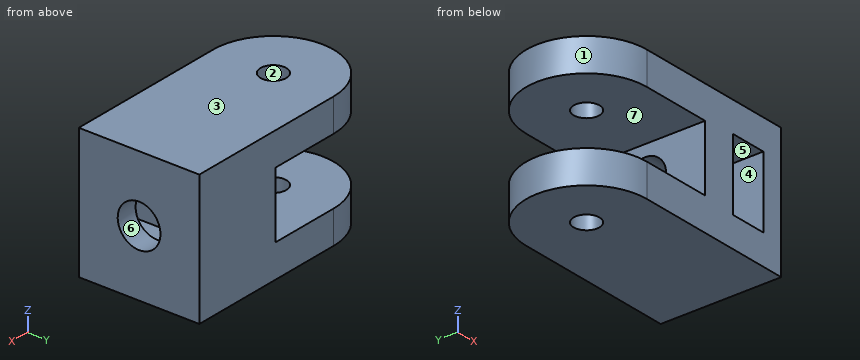
```python
from build123d import *

# Parameters (mm, degrees)
BOSS_EXTRUDE1_DEPTH            = 24
SKETCH2_W                      = 30.110806601
SKETCH2_H                      = 12
CUT_EXTRUDE1_DEPTH             = 45.271887242
CUT_EXTRUDE2_DEPTH             = 6.8
F_7_8_7_8_DIAMETER_HOLE1_D     = 7.8
F_7_8_7_8_DIAMETER_HOLE1_DEPTH = 6.2
F_7_8_7_8_DIAMETER_HOLE2_D     = 7.8
F_4_7_4_7_DIAMETER_HOLE1_D     = 4.7
F_4_7_4_7_DIAMETER_HOLE1_DEPTH = 6
F_4_7_4_7_DIAMETER_HOLE2_D     = 4.7


with BuildPart() as part:
    # Sketch1 → Boss-Extrude1 (new body)
    with BuildSketch(Plane(origin=(0, 0, -24), x_dir=(-1, 0, 0), z_dir=(0, 0, -1))):
        with BuildLine():
            Line((0, 11), (-30, 11))
            Line((-30, 11), (-30, -11))
            Line((-30, -11), (0, -11))
            ThreePointArc((0, -11), (11, 0), (0, 11))
        make_face()
    extrude(amount=-BOSS_EXTRUDE1_DEPTH)

    # Sketch2 → Cut-Extrude1 (cut, through all)
    with BuildSketch(Plane(origin=(0, 11, 0), x_dir=(-1, 0, 0), z_dir=(0, 1, 0))):
        with Locations((2.055403301, -12)):
            Rectangle(SKETCH2_W, SKETCH2_H)
    extrude(amount=-CUT_EXTRUDE1_DEPTH, mode=Mode.SUBTRACT)

    # Sketch3 → Cut-Extrude2 (cut)
    with BuildSketch(Plane(origin=(19.2, 0, 0), x_dir=(0, -1, 0), z_dir=(-1, 0, 0))):
        Polygon((11, -18.5), (11, -5.5), (-3.75277675, -5.5), (-7.505553499, -12), (-3.75277675, -18.5), align=None)
    extrude(amount=-CUT_EXTRUDE2_DEPTH, mode=Mode.SUBTRACT)

    # Ø7.8 (7.8) Diameter Hole1
    with Locations(Plane.ZY.offset(-13)):
        with Locations((-12, 0)):
            Hole(F_7_8_7_8_DIAMETER_HOLE1_D / 2, depth=F_7_8_7_8_DIAMETER_HOLE1_DEPTH)

    # Ø7.8 (7.8) Diameter Hole2 (through all)
    with Locations(Plane.ZY.offset(-26)):
        with Locations((-12, 0)):
            Hole(F_7_8_7_8_DIAMETER_HOLE2_D / 2)

    # Ø4.7 (4.7) Diameter Hole1
    with Locations(Plane(origin=(0, 0, -24), x_dir=(-1, 0, 0), z_dir=(0, 0, -1))):
        with Locations((0, 0)):
            Hole(F_4_7_4_7_DIAMETER_HOLE1_D / 2, depth=F_4_7_4_7_DIAMETER_HOLE1_DEPTH)

    # Ø4.7 (4.7) Diameter Hole2 (through all)
    with Locations(Plane(origin=(0, 0, -6), x_dir=(-1, 0, 0), z_dir=(0, 0, -1))):
        with Locations((0, 0)):
            Hole(F_4_7_4_7_DIAMETER_HOLE2_D / 2)


solid = part.part
```
The model under review builds one solid part; all positions refer to its coordinate system, in mm. Face numbers are marked on the shaded views. A direction names the side the tool comes from. Coordinates: 2 decimals unless noted, no trailing zeros. Write each loop counter-clockwise with the first axis right and the second up, starting at its lowest first coordinate (ties: lowest second). Pieces come first, ordered by that corner, then holes. Notation, with made-up numbers: (14, -22) -> (38, -22) arc R19 cw to (38, 7) -> close; hole circle Ø11 at (1, 36.25). An arc over 180 degrees is marked (long way). One line per item, written item: value. Start each with the question number.
Q1. For the marked faces 5, 6 and 7, list the 3-axis set-ups (+Z, -Z, +X, -X, +Y, -Y) from which the entire face can be reached by the end or side of a thin tool; tool diameter is ignored.
Q2. Add section A-A, the plane y = 0. Give the boundary of the cut face in (x, z), then the cut area to 3 significant figures.
Q3. The part is to be moulded in two halves that separate along X. For the marked faces 1, 2, 3 and 4, say which applies: +X half, -X half, draft (parallel to the pull), parting line (faces both ways), or undercut.
Q4. Add section D-D, the plane z = -14.75. Give the boundary of the cut face in (x, y), then the cut area to 3 significant figures.
Q5. Add section C-C, the plane y = -3.25. Give the boundary of the cut face in (x, z).
Q6. Add section B-B, the plane x = 10. Give the boundary of the cut face in (y, z).
Q7. To check wall thickness, follow probe 1 along X at (y, z) = (-6.5, -8.5); probe 2 along Z at (x, y) = (11.5, -5.75); probe 3 along Y at (x, z) = (28, -12). State the ranges of each line that lie inside material, in increasing order.
Q8. Clearance check with a flat-ended pin moving along its axis: P1, Ø4, axis at y = 1.5, z = -8.5, coming from the -X side. State where the tip first meets the part, or that it passes through.
Response:
1. face 5: -Y
1. face 6: +X, -X
1. face 7: -X, +Y, -Y
2. outline: (-11, -24) -> (-2.35, -24) -> (-2.35, -18) -> (-11, -18) -> close; (-11, -6) -> (-2.35, -6) -> (-2.35, 0) -> (-11, 0) -> close; (2.35, -24) -> (30, -24) -> (30, -15.9) -> (26, -15.9) -> (26, -18.5) -> (19.2, -18.5) -> (19.2, -15.9) -> (13, -15.9) -> (13, -18) -> (2.35, -18) -> close; (2.35, -6) -> (13, -6) -> (13, -8.1) -> (19.2, -8.1) -> (19.2, -5.5) -> (26, -5.5) -> (26, -8.1) -> (30, -8.1) -> (30, 0) -> (2.35, 0) -> close
2. area: 472 mm²
3. face 1: -X half
3. face 2: undercut
3. face 3: draft
3. face 4: undercut
4. outline: (13, -11) -> (19.2, -11) -> (19.2, -2.77) -> (13, -2.77) -> close; (13, 2.77) -> (19.2, 2.77) -> (19.2, 5.92) -> (26, 5.92) -> (26, 2.77) -> (30, 2.77) -> (30, 11) -> (13, 11) -> close; (26, -11) -> (30, -11) -> (30, -2.77) -> (26, -2.77) -> close
4. area: 203 mm²
5. outline: (-10.51, -24) -> (30, -24) -> (30, -14.16) -> (26, -14.16) -> (26, -18.5) -> (19.2, -18.5) -> (19.2, -14.16) -> (13, -14.16) -> (13, -18) -> (-10.51, -18) -> close; (-10.51, -6) -> (13, -6) -> (13, -9.84) -> (19.2, -9.84) -> (19.2, -5.5) -> (26, -5.5) -> (26, -9.84) -> (30, -9.84) -> (30, 0) -> (-10.51, 0) -> close
6. outline: (-11, -24) -> (11, -24) -> (11, -18) -> (-11, -18) -> close; (-11, -6) -> (11, -6) -> (11, 0) -> (-11, 0) -> close
7. probe 1: 13 to 19.2, 26 to 30
7. probe 2: -24 to -18, -6 to 0
7. probe 3: -11 to -3.9, 3.9 to 11
8. P1: x = 13
